Verification items for this drawing (mm, ordinates from the low corner). A direction names the side the tool comes from. Round coordinates to 2 decimals unless told otherwise and drop trailing zeros. Order: outer loops, then holes, each group sorted by start corner. A loop starts at its lowest first (then second) coordinate and runs counter-clockwise, first axis right, second up. Notation, with made-up numbers: M -13.5,-21.75 L 10.5,-21.75 A16 cw 10.5,-13.75 Z; hole C -12.75,54 d5. An arc over 180 degrees is marked long. Return JSON: item names as keys, results as strings. Group by question number.
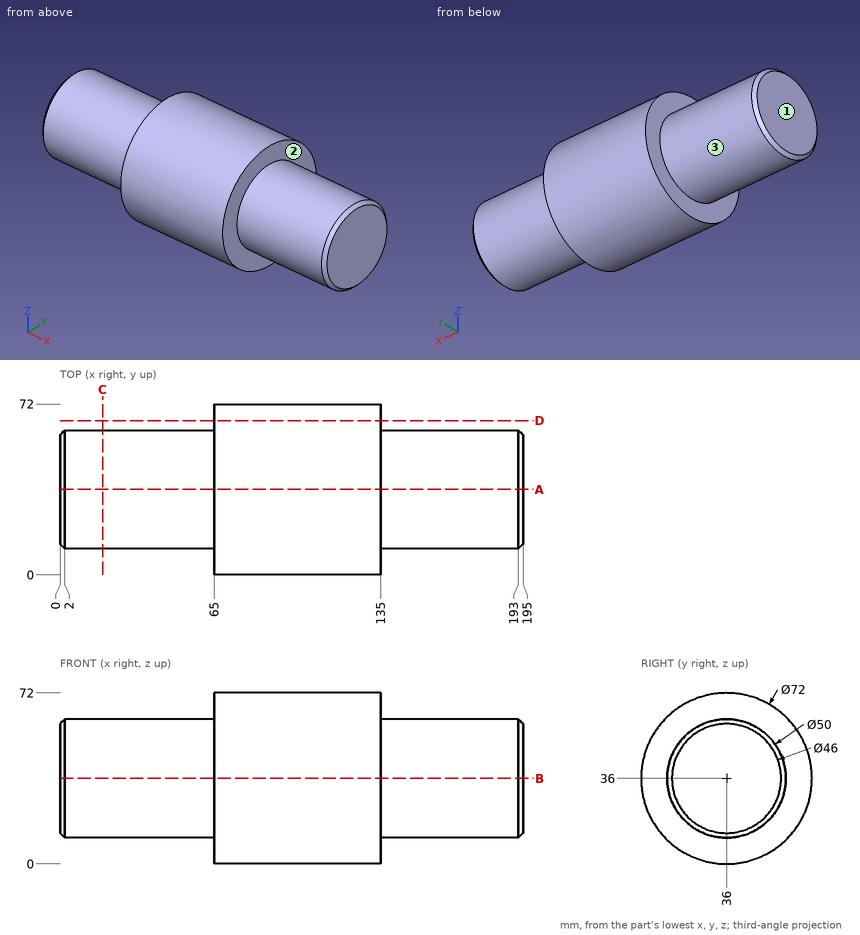
1. Cross-section at D-D (y = 65). Enter the section's corners in (x, z).
2. Access from +Z, -Z, +X, -X, +Y, -Y to the whole of each face (thin tool, end or side, straight path). Record for the marked faces 1, 2 and 3.
3. Thickness scan on line 1 along X through (y, z) = (9.5, 20); line 2 along X through (y, z) = (49.5, 15); line 3 along Y through (x, z) = (45.5, 23). Record the ranges inside material, lowest first. Write a range as from..to.
4. Go/stop test with flat-tipped pins: pin 1 (5 mm diameter, centred on x = 68, z = 9, fed in from +Y); pin 2 (1.5 mm diameter, centred on x = 68.5, z = 53.5, fed in from +Y); pin 3 (1 mm diameter, centred on x = 166.5, y = 17.5, fed in from -Z). Record where each tip stops, or that it passes through.
5. Cross-section at C-C (x = 18). Enter the section's corners in (y, z).
6. Cross-section at A-A (y = 36). Enter the section's corners in (x, z), plus the area to 3 significant figures.
Computed:
{
 "1": {"outline": "M 65,14.67 L 135,14.67 L 135,57.33 L 65,57.33 Z"},
 "2": {"face 1": "+Z, -Z, -X, +Y, -Y", "face 2": "+X", "face 3": "-X"},
 "3": {"line 1": "x = 65..135", "line 2": "x = 1.96..193.04", "line 3": "y = 14.65..57.35"},
 "4": {"pin 1": "stops at y = 62.38", "pin 2": "stops at y = 67.87", "pin 3": "stops at z = 18.65"},
 "5": {"outline": "C 36,36 d50"},
 "6": {"outline": "M 0,13 L 2,11 L 65,11 L 65,0 L 135,0 L 135,11 L 193,11 L 195,13 L 195,59 L 193,61 L 135,61 L 135,72 L 65,72 L 65,61 L 2,61 L 0,59 Z", "area": "11,300 mm²"}
}
